from build123d import *

# Parameters (mm, degrees)
F1_DEPTH = 24
F2_R     = 1.5
F3_DEPTH = 25
F4_R     = 0.5


with BuildPart() as f1:
    # F0 (on Top) → F1 (new body)
    with BuildSketch(Plane.XY):
        Polygon((-15.5, 0), (0, 0), (15.5, 0), (15.5, 18.5), (28.5, 18.5), (28.5, 0), (37.5, 0), (37.5, 2), (30.5, 2), (30.5, 18.5), (37.5, 18.5), (37.5, 20.5), (13.5, 20.5), (13.5, 2), (0, 2), (-13.5, 2), (-13.5, 20.5), (-37.5, 20.5), (-37.5, 18.5), (-30.5, 18.5), (-30.5, 2), (-37.5, 2), (-37.5, 0), (-28.5, 0), (-28.5, 18.5), (-15.5, 18.5), align=None)
    extrude(amount=F1_DEPTH)

    # F2 (on face) → F3 (cut)
    with BuildSketch(Plane.XZ):
        with Locations((-33.5, 12)):
            Circle(F2_R)
        with Locations((0, 12)):
            Circle(F2_R)
        with Locations((33.5, 12)):
            Circle(F2_R)
    extrude(amount=-F3_DEPTH, mode=Mode.SUBTRACT)

    # F4
    f4_edges = [f1.edges().sort_by_distance(p)[0] for p in [
        (-13.5, 20.5, 12),
        (13.5, 20.5, 12),
        (15.5, 0, 12),
        (-28.5, 0, 12),
        (-15.5, 0, 12),
        (28.5, 0, 12),
        (37.5, 20.5, 12),
        (37.5, 18.5, 12),
        (37.5, 2, 12),
        (37.5, 0, 12),
        (-37.5, 20.5, 12),
        (-37.5, 18.5, 12),
        (-37.5, 2, 12),
        (-37.5, 0, 12),
    ]]
    fillet(f4_edges, radius=F4_R)


solid = f1.part
Verification items for the finished model (mm, model axes). A direction names the side the tool comes from. Coordinates: 2 decimals unless noted, no trailing zeros. Order: outer loops, then holes, each group sorted by start corner. A loop starts at its lowest first (then second) coordinate and runs counter-clockwise, first axis right, second up.
Item 1: Section check A-A, the plane y = 5.75. Enter the section's corners in (x, z).
Filled in:
outline: (-30.5, 0) - (-28.5, 0) - (-28.5, 24) - (-30.5, 24) - close; (-15.5, 0) - (-13.5, 0) - (-13.5, 24) - (-15.5, 24) - close; (13.5, 0) - (15.5, 0) - (15.5, 24) - (13.5, 24) - close; (28.5, 0) - (30.5, 0) - (30.5, 24) - (28.5, 24) - close
Item 2: Material ranges on L1, parallel to X at y = 6.25, z = 1.5; L2, parallel to Z at x = -33.5, y = 1.45; L3, parallel to Y at x = -1, z = 17, recorded low to high.
Filled in:
L1: x = -30.5 to -28.5, -15.5 to -13.5, 13.5 to 15.5, 28.5 to 30.5
L2: z = 0 to 10.5, 13.5 to 24
L3: y = 0 to 2
Item 3: Release check for a two-part mould opening along X. For faces 1 (the face through (15.5, 9, 12)), 2 (the face through (30.5, 10, 12)), 3 (the face through (3, 1, 24)) record: +X half, -X half, draft (parallel to the pull), parting line (faces both ways), or undercut.
Filled in:
face 1: undercut
face 2: +X half
face 3: draft
Item 4: Access from +Z, -Z, +X, -X, +Y, -Y to the whole of each face (thin tool, end or side, straight path). Record for faces 4 (the face through (35.15, 18.5, 11.83)), 5 (the face through (-13.5, 11, 12)), 6 (the face through (28.5, 10, 12)), 7 (the face through (-35.15, 2, 11.83)), 8 (the face through (3, 1, 0)).
Filled in:
face 4: +Z, -Z, +X
face 5: +Z, -Z, +Y
face 6: +Z, -Z, -Y
face 7: +Z, -Z, -X
face 8: -Z, +X, -X, +Y, -Y
Item 5: Depth check by flat-ended pin: pin 1 (4 mm diameter, centred on x = -25, z = 11.5, fed in from -Y); pin 2 (5.5 mm diameter, centred on y = 10.5, z = 11.5, fed in from +X); pin 3 (7 mm diameter, centred on x = 2.5, z = 14, fed in from +Y). Enter the tip coordinate at first touch or a pass-through.
Filled in:
pin 1: stops at y = 18.5
pin 2: stops at x = 30.5
pin 3: stops at y = 2
Item 6: Section check C-C, the plane z = 12. Give the number of separate pieces and of enclosed holes in the cut face, then the cut area to 3 significant figures.
Filled in:
separate pieces: 6
enclosed holes: 0
area: 295 mm2
Item 7: Section check B-B, the plane x = -33.5. Enter the section's corners in (y, z), then the cut area to 3 significant figures.
Filled in:
outline: (0, 0) - (2, 0) - (2, 10.5) - (0, 10.5) - close; (0, 13.5) - (2, 13.5) - (2, 24) - (0, 24) - close; (18.5, 0) - (20.5, 0) - (20.5, 10.5) - (18.5, 10.5) - close; (18.5, 13.5) - (20.5, 13.5) - (20.5, 24) - (18.5, 24) - close
area: 84.0 mm2
